```python
from build123d import *

# Parameters (mm, degrees)
SKETCH2_W           = 257.3
SKETCH2_H           = 327.9
BOSS_EXTRUDE1_DEPTH = 120
CUT_EXTRUDE1_DEPTH  = 330
CUT_EXTRUDE2_DEPTH  = 425
SKETCH5_R           = 6
CUT_EXTRUDE3_DEPTH  = 21


with BuildPart() as part:
    # Sketch2 → Boss-Extrude1 (new body)
    with BuildSketch(Plane(origin=(0, 0, 0), x_dir=(1, 0, 0), z_dir=(0, 1, 0))):
        Rectangle(SKETCH2_W, SKETCH2_H)
    extrude(amount=BOSS_EXTRUDE1_DEPTH)

    # Sketch3 → Cut-Extrude1 (cut)
    with BuildSketch(Plane.XY.offset(163.95)):
        Polygon((128.65, 0), (-128.65, 120), (128.65, 120), align=None)
    extrude(amount=-CUT_EXTRUDE1_DEPTH, mode=Mode.SUBTRACT)

    # Sketch4 → Cut-Extrude2 (cut)
    with BuildSketch(Plane.XY.offset(163.95)):
        Polygon((-114.703132504, 94.894537232), (-114.703132504, 12.894537232), (61.096867496, 12.894537232), align=None)
    extrude(amount=-CUT_EXTRUDE2_DEPTH, mode=Mode.SUBTRACT)

    # Sketch5 → Cut-Extrude3 (cut)
    with BuildSketch(Plane.ZY.offset(128.65)):
        with Locations((-114.05, 80)):
            Circle(SKETCH5_R)
        with Locations((-114.05, 26.7)):
            Circle(SKETCH5_R)
        with Locations((113.95, 80)):
            Circle(SKETCH5_R)
        with Locations((113.95, 26.7)):
            Circle(SKETCH5_R)
    extrude(amount=-CUT_EXTRUDE3_DEPTH, mode=Mode.SUBTRACT)


solid = part.part
```
Could you check a few things on this model? Use its own coordinates, in mm. A direction names the side the tool comes from. Round coordinates to 2 decimals unless told otherwise and drop trailing zeros. Loops run counter-clockwise (first coordinate to the right, second up) from the corner with the lowest first, then second, coordinate; pieces in that order, holes last. Notation, with made-up numbers: (49.5, 52.5) - (70.5, 52.5) arc R11 cw to (70.5, 61.5) - close; hole circle Ø9 at (15.25, 50.25). An arc over 180 degrees is marked (long way). Use CSV: the item, a comma, the result in double quotes.
Item 1: I need wall thicknesses on L1, parallel to Z at x = -117, y = 26; L2, parallel to Y at x = -125, z = 113; L3, parallel to Y at x = -117.75, z = 113.95. Which ranges of each line are inside material? Lowest first, please. Write a range as [from, to].
Here are the results:
L1,"z = [-163.95, -120.01], [-108.09, 107.99], [119.91, 163.95]"
L2,"y = [0, 20.78], [32.62, 74.08], [85.92, 118.3]"
L3,"y = [0, 20.7], [32.7, 74], [86, 114.92]"
Item 2: If we section it at A-A on z = -114.05: List the corners of the cut face in (x, y) for me, then the cut area to 3 significant figures.
Here are the results:
outline,"(-128.65, 0) - (128.65, 0) - (-128.65, 120) - (-128.65, 86) - (-114.7, 86) - (-114.7, 94.89) - (61.1, 12.89) - (-114.7, 12.89) - (-114.7, 20.7) - (-128.65, 20.7) - close; (-128.65, 32.7) - (-114.7, 32.7) - (-114.7, 74) - (-128.65, 74) - close"
area,"7,900 mm²"
Item 3: If we section it at C-C on x = -110.5: List the corners of the cut face in (y, z) for me.
Here are the results:
outline,"(0, -163.95) - (12.89, -163.95) - (12.89, 163.95) - (0, 163.95) - close; (92.93, -163.95) - (111.54, -163.95) - (111.54, 163.95) - (92.93, 163.95) - close"
Item 4: Will these pins go through, and if not, where does the flat tip stop? pin 1 (15.5 mm diameter, centred on y = 80, z = 113.95, fed in from +X); pin 2 (3 mm diameter, centred on x = 40.5, z = 105, fed in from +Y); pin 3 (19 mm diameter, centred on y = 26.7, z = -114.05, fed in from +X); pin 4 (19 mm diameter, centred on y = 80, z = -114.05, fed in from -X).
Here are the results:
pin 1,"stops at x = -26.27"
pin 2,"stops at y = 41.81"
pin 3,"stops at x = 91.77"
pin 4,"stops at x = -128.65"
Item 5: If we mould it in two halves opening along Y, with no side actions, what happens to faces 1 (the flat face through (-30, 59, 163.95)), 2 (the flat face through (1.8, 59.16, 2.3)), 3 (the cylindrical face through (-121.774, 28.502, -108.327))? For each: pulls with the +Y half, pulls with the -Y half, needs draft (parallel to the pull), parting line crosses it, or undercut.
Here are the results:
face 1,"needs draft"
face 2,"pulls with the +Y half"
face 3,"undercut"
Item 6: If we section it at B-B on y = 91: List the corners of the cut face in (x, z) for me, then the cut area to 3 significant figures.
Here are the results:
outline,"(-128.65, -163.95) - (-114.7, -163.95) - (-114.7, 163.95) - (-128.65, 163.95) - close; (-106.35, -163.95) - (-66.47, -163.95) - (-66.47, 163.95) - (-106.35, 163.95) - close"
area,"17,700 mm²"
Item 7: For faces 4 (the flat face through (-28, 12.895, 2)), 5 (the flat face through (-2, 0, -2)), 6 (the cylindrical face through (-121.774, 28.502, 119.673)), which set-ups out of +Z, -Z, +X, -X, +Y, -Y let a thin tool reach every point of the face, with its end or its side?
Here are the results:
face 4,"+Z, -Z"
face 5,"+Z, -Z, +X, -X, -Y"
face 6,"-X"
Item 8: If we section it at D-D on y = 26.7: List the corners of the cut face in (x, z) for me, then the cut area to 3 significant figures.
Here are the results:
outline,"(-128.65, -163.95) - (-114.7, -163.95) - (-114.7, -120.05) - (-128.65, -120.05) - close; (-128.65, -108.05) - (-114.7, -108.05) - (-114.7, 107.95) - (-128.65, 107.95) - close; (-128.65, 119.95) - (-114.7, 119.95) - (-114.7, 163.95) - (-128.65, 163.95) - close; (31.5, -163.95) - (71.4, -163.95) - (71.4, 163.95) - (31.5, 163.95) - close"
area,"17,300 mm²"
